```python
from build123d import *

# Parameters (mm, degrees)
SZKIC2_R = 3


with BuildPart() as part:
    # Wyciągnięcie po ścieżce1: sweep along a path in Szkic1
    with BuildLine(Plane(origin=(0, 0, 0), x_dir=(1, 0, 0), z_dir=(0, 1, 0))) as wyci_gni_cie_po_cie_ce1_path:
        Line((-60, -25), (-60, -20))
        ThreePointArc((-60, -20), (-58.535533906, -16.464466094), (-55, -15))
        Line((-55, -15), (-35, -15))
        ThreePointArc((-35, -15), (-31.464466094, -16.464466094), (-30, -20))
        Line((-30, -20), (-30, -25))
    # Szkic2 → Wyciągnięcie po ścieżce1 (sweep)
    with BuildSketch(Plane(origin=(-60, 0, 25), x_dir=(-1, 0, 0), z_dir=(0, 0, -1))):
        Circle(SZKIC2_R)
    sweep(path=wyci_gni_cie_po_cie_ce1_path.line)


solid = part.part
```
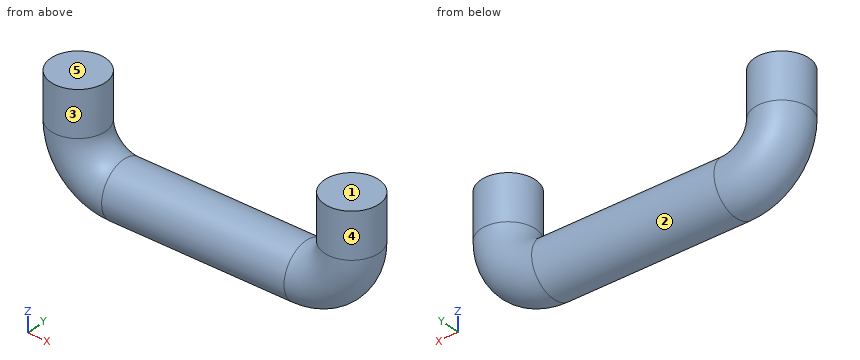
Input: part model. Units: mm. Frame: model coordinates. Face numbers are marked on the shaded views. A direction names the side the tool comes from. Round coordinates to 2 decimals unless told otherwise and drop trailing zeros. Loops run counter-clockwise (first coordinate to the right, second up) from the corner with the lowest first, then second, coordinate; pieces in that order, holes last. Notation, with made-up numbers: (89.25, 89.5) -> (123.25, 89.5) arc R24 cw to (123.25, 105.5) -> close; hole circle Ø4 at (45, -35). An arc over 180 degrees is marked (long way). Use one line per item in the form item = value. Start each with the question number.
Item 1: Section query C-C on x = -50. Return the cut outline in (y, z).
Item 2: Section query B-B on z = 23.5. Return the cut outline in (x, y).
Item 3: Set-up query: the marked faces 1 and 2. Return all of +Z, -Z, +X, -X, +Y, -Y with unobstructed straight access to the full face (end or side cutting, diameter ignored); none if empty.
Item 4: Section query A-A on y = 0. Return the cut outline in (x, z), then the cut area to 3 significant figures.
Item 5: Section query D-D on y = 1.75. Return the cut outline in (x, z).
Item 6: Mould query, pull axis X, two halves, no side actions, for the marked faces 3, 4 and 5. Classes: pulls with the +X half, pulls with the -X half, needs draft (parallel to the pull), parting line crosses it, or undercut.
Item 7: Contact query for flat-ended pins moving along their axis: pin 1 Ø1 at (x, z) = (-50.5, 18) entering from -Y; pin 2 Ø1 at (y, z) = (1, 20) entering from -X; pin 3 Ø2 at (y, z) = (1, 21) entering from +X; pin 4 Ø1.5 at (x, y) = (-45.5, -2.5) entering from +Z. Output: stop coordinate, or through.
Item 8: Material intervals for L1, parallel to X at y = 2.75, z = 21.75; L2, parallel to X at y = -1, z = 18; L3, parallel to Y at x = -61, z = 22.75, sorted ascending. Write a range as from..to.
Ans:
q1.outline = circle Ø6 at (0, 15)
q2.outline = circle Ø6 at (-60, 0); circle Ø6 at (-30, 0)
q3.face_1 = +Z, +X, -X, +Y, -Y
q3.face_2 = none
q4.outline = (-63, 20) arc R8 ccw to (-55, 12) -> (-35, 12) arc R8 ccw to (-27, 20) -> (-27, 25) -> (-33, 25) -> (-33, 20) arc R2 cw to (-35, 18) -> (-55, 18) arc R2 cw to (-57, 20) -> (-57, 25) -> (-63, 25) -> close
q4.area = 274 mm^2
q5.outline = (-62.44, 20) arc R7.44 ccw to (-55, 12.56) -> (-35, 12.56) arc R7.44 ccw to (-27.56, 20) -> (-27.56, 25) -> (-32.44, 25) -> (-32.44, 20) arc R2.56 cw to (-35, 17.44) -> (-55, 17.44) arc R2.56 cw to (-57.56, 20) -> (-57.56, 25) -> (-62.44, 25) -> close
q6.face_3 = undercut
q6.face_4 = undercut
q6.face_5 = needs draft
q7.pin_1 = -1.66
q7.pin_2 = -62.96
q7.pin_3 = -27
q7.pin_4 = 17.44
q8.L1 = -61.2..-58.8, -31.2..-28.8
q8.L2 = -62.57..-55.85, -34.15..-27.43
q8.L3 = -2.83..2.83
